Autodesk Inventor part; units mm, degrees
ref_plane "YZ Plane" through (0, 0, 0) normal (1, 0, 0) x (0, 1, 0)
ref_plane "XZ Plane" through (0, 0, 0) normal (0, 1, 0) x (-1, 0, 0)
ref_plane "XY Plane" through (0, 0, 0) normal (0, 0, 1) x (1, 0, 0)
sketch "Sketch1" plane through (0, 0, 0) normal (0, 0, 1) x (1, 0, 0)
  line L0 (0, 24.2) -> (54.2, 24.2)
  line L1 (54.2, 24.2) -> (54.2, 0)
  line L2 (54.2, 0) -> (0, 0)
  line L3 (0, 0) -> (0, 24.2)
  circle A0 centre (44.95, 21.7) radius 1.5
  circle A1 centre (8.6, 2.5) radius 1.5
  dimension "d0" = 54.2
  dimension "d1" = 24.2
  dimension "d2" = 3
  dimension "d3" = 2.5
  dimension "d4" = 9.25
  dimension "d5" = 2.5
  dimension "d6" = 8.6
extrude "Extrusion1" add sketch "Sketch1" along normal blind 1.6
properties part number "XL4015"
Here's how the part is built. I have some questions about the finished solid (model axes, mm). Round coordinates to 2 decimals unless told otherwise and drop trailing zeros. Order: outer loops, then holes, each group sorted by start corner. A loop starts at its lowest first (then second) coordinate and runs counter-clockwise, first axis right, second up. Notation, with made-up numbers: M 2,2 L 15,2 A24 cw 15,27 Z; hole C 67.5,53.25 d7. An arc over 180 degrees is marked long. Answer in a Markdown table with one row per item.
Item 1: If I drill on L1, parallel to Y at x = 8.6, z = 1.25; L2, parallel to Y at x = 44.95, z = 1.2; L3, parallel to X at y = 21.5, z = 0.7, over which ranges is the centre line in solid material (lowest first)? Write a range as from..to.
A:
| item | result |
|---|---|
| L1 | y = 0..1, 4..24.2 |
| L2 | y = 0..20.2, 23.2..24.2 |
| L3 | x = 0..43.46, 46.44..54.2 |
Item 2: Imagine slicing it at B-B, the plane y = 2.5. Write out the boundary of the cut face in (x, z), and give its area (3 significant figures).
A:
| item | result |
|---|---|
| outline | M 0,0 L 7.1,0 L 7.1,1.6 L 0,1.6 Z; M 10.1,0 L 54.2,0 L 54.2,1.6 L 10.1,1.6 Z |
| area | 81.9 mm2 |
Item 3: Imagine slicing it at A-A, the plane x = 8.6. Write out the boundary of the cut face in (y, z), and give its area (3 significant figures).
A:
| item | result |
|---|---|
| outline | M 0,0 L 1,0 L 1,1.6 L 0,1.6 Z; M 4,0 L 24.2,0 L 24.2,1.6 L 4,1.6 Z |
| area | 33.9 mm2 |
Item 4: I'm going to push a flat-ended pin straight in: pin 1 (2.5 mm diameter, centred on x = 8.6, y = 2.5, fed in from -Z). Where does the tip first touch, or does it pass through?
A:
| item | result |
|---|---|
| pin 1 | passes through |
